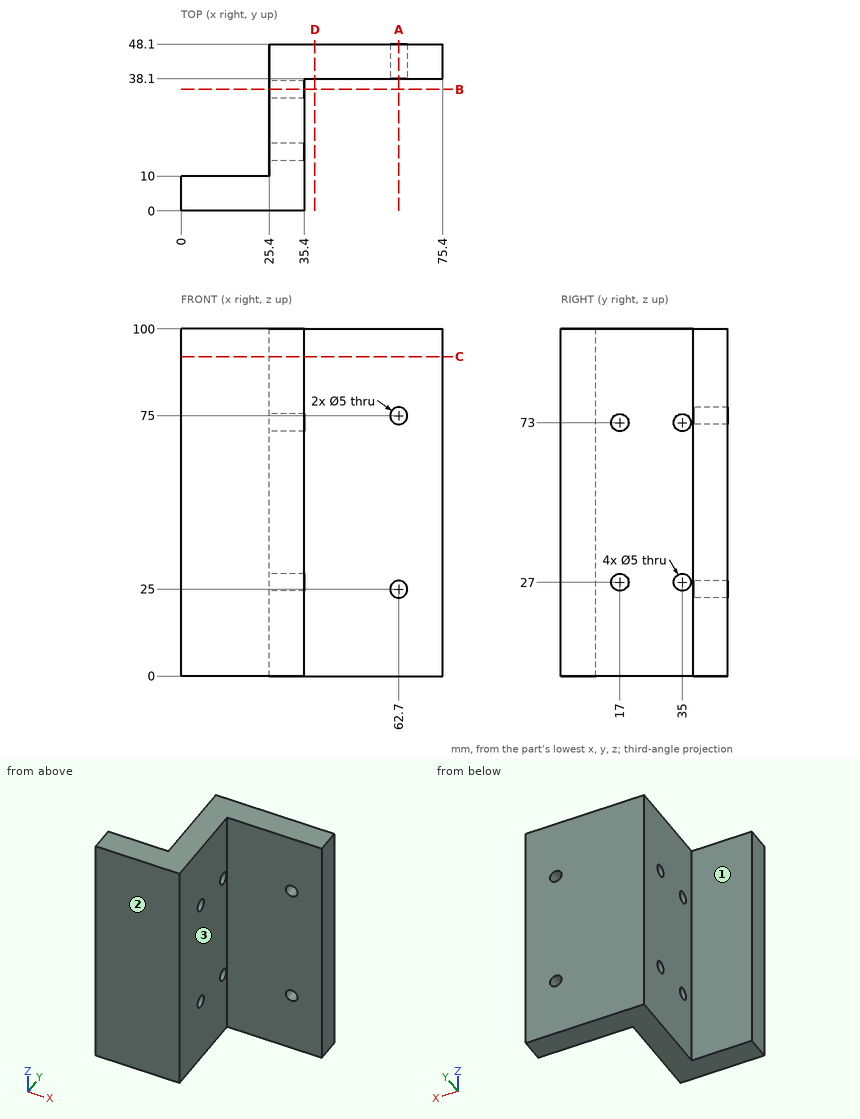
Here's the drawing with two shaded views (mm, measured from the low corner). I have some questions. A direction names the side the tool comes from. Coordinates: 2 decimals unless noted, no trailing zeros. Loops run counter-clockwise (first coordinate to the right, second up) from the corner with the lowest first, then second, coordinate; pieces in that order, holes last. Notation, with made-up numbers: (-11, -1.5) -> (39, -1.5) arc R28 ccw to (39, 34.5) -> close; hole circle Ø7 at (-16, 82.25). An arc over 180 degrees is marked (long way). Answer as a JSON object with one key per item and string values.
1) If I drill on line 1 (Z direction, x = 62.7, y = 41); line 2 (Y direction, x = 32, z = 27); line 3 (Z direction, x = 62, y = 40), over which ranges is the centre line in solid material (lowest first)?
Results:
{"line 1": "z = 0 to 22.5, 27.5 to 72.5, 77.5 to 100", "line 2": "y = 0 to 14.5, 19.5 to 32.5, 37.5 to 48.1", "line 3": "z = 0 to 22.6, 27.4 to 72.6, 77.4 to 100"}
2) Imagine slicing it at D-D (x = 38.5). Please give me the cut outline in (y, z).
Results:
{"outline": "(38.1, 0) -> (48.1, 0) -> (48.1, 100) -> (38.1, 100) -> close"}
3) For the marked faces 1, 2 and 3, which set-ups out of +Z, -Z, +X, -X, +Y, -Y let a thin tool reach every point of the face, with its end or its side?
Results:
{"face 1": "+Z, -Z, -X, +Y", "face 2": "+Z, -Z, +X, -X, -Y", "face 3": "+Z, -Z, +X, -Y"}
4) For P1, Ø20.5, axis at x = 11, z = 56, coming from the +Y side; P2, Ø6.5, axis at y = 17, z = 73, coming from the -X side; P3, Ø10, axis at x = 63, z = 76, coming from the -Y side, each with a flat end and sliding along its axis, tell me the tip position at first contact or that it passes through.
Results:
{"P1": "stops at y = 10", "P2": "stops at x = 25.4", "P3": "stops at y = 38.1"}
5) Imagine slicing it at B-B (y = 35). Please give me the cut outline in (x, z), then the cut area to 3 significant figures.
Results:
{"outline": "(25.4, 0) -> (35.4, 0) -> (35.4, 24.5) -> (25.4, 24.5) -> close; (25.4, 29.5) -> (35.4, 29.5) -> (35.4, 70.5) -> (25.4, 70.5) -> close; (25.4, 75.5) -> (35.4, 75.5) -> (35.4, 100) -> (25.4, 100) -> close", "area": "900 mm^2"}
6) Imagine slicing it at C-C (z = 92). Please give me the cut outline in (x, y).
Results:
{"outline": "(0, 0) -> (35.4, 0) -> (35.4, 38.1) -> (75.4, 38.1) -> (75.4, 48.1) -> (25.4, 48.1) -> (25.4, 10) -> (0, 10) -> close"}
7) Imagine slicing it at A-A (x = 62.7). Please give me the cut outline in (y, z), then the cut area to 3 significant figures.
Results:
{"outline": "(38.1, 0) -> (48.1, 0) -> (48.1, 22.5) -> (38.1, 22.5) -> close; (38.1, 27.5) -> (48.1, 27.5) -> (48.1, 72.5) -> (38.1, 72.5) -> close; (38.1, 77.5) -> (48.1, 77.5) -> (48.1, 100) -> (38.1, 100) -> close", "area": "900 mm^2"}
